from build123d import *

# Parameters (mm, degrees)
F0_W          = 152.4
F0_H          = 15.24
F1_DEPTH      = 12.7
F2_T1_DEPTH   = 190.5
F4_W          = 25.0697992742
F4_H          = 11.7348134518
F5_DEPTH      = 12.7
F5_DEPTH_BACK = 12.7
F7_DEPTH      = 7.62
F7_DEPTH_BACK = 7.62
F8_W          = 65.6082034111
F8_H          = 914.4
F9_DEPTH      = 5.08
F9_DEPTH_BACK = 5.08
F11_DEPTH     = 914.4
F12_DEPTH     = 12.7
F16_R         = 5.08


# Not quite as in the source:
# - a fillet or chamfer that OpenCascade refuses, or shapes differently, is made with other operations: its cross-section is extruded or revolved along the edge and cut away or added


with BuildPart() as f1:
    # F0 (on Right) → F1 (new body)
    with BuildSketch(Plane.YZ):
        with Locations((76.2, -7.62)):
            Rectangle(F0_W, F0_H)
    extrude(amount=F1_DEPTH)

    # F2: fillet of radius 7.62 on 4 edges, made by hand

    # F2_s2 → F2_t1 (cut)
    with BuildSketch(Plane.XZ.offset(-171.45)):
        with BuildLine():
            ThreePointArc((7.62, 0), (2.2318463274, -2.2318463274), (0, -7.62))
            Line((0, -7.62), (0, 0))
            Line((0, 0), (7.62, 0))
        make_face()
        with BuildLine():
            ThreePointArc((7.62, -15.24), (2.2318463274, -13.0081536726), (0, -7.62))
            Line((0, -7.62), (0, -15.24))
            Line((0, -15.24), (7.62, -15.24))
        make_face()
        with BuildLine():
            ThreePointArc((5.08, 0), (10.4681536726, -2.2318463274), (12.7, -7.62))
            Line((12.7, -7.62), (12.7, 0))
            Line((12.7, 0), (5.08, 0))
        make_face()
        with BuildLine():
            ThreePointArc((5.08, -15.24), (10.4681536726, -13.0081536726), (12.7, -7.62))
            Line((12.7, -7.62), (12.7, -15.24))
            Line((12.7, -15.24), (5.08, -15.24))
        make_face()
    extrude(amount=F2_T1_DEPTH, mode=Mode.SUBTRACT)

    # F4 (on offset) → F5 (join, two sides)
    with BuildSketch(Plane.XY.offset(-7.62)) as f5_sk:
        with Locations((6.0101542622, 157.924503088)):
            Rectangle(F4_W, F4_H)
    extrude(amount=F5_DEPTH)
    extrude(f5_sk.sketch, amount=-F5_DEPTH_BACK)

    # F6 (on offset) → F7 (join, two sides)
    with BuildSketch(Plane.XY.offset(-7.62)) as f7_sk:
        with BuildLine():
            Line((6.3893780661, -0.6641601572), (12.5797659928, -0.6641601572))
            ThreePointArc((12.5797659928, -0.6641601572), (34.2227463889, 6.8879561013), (46.4923181534, 26.2505661817))
            Line((46.4923181534, 26.2505661817), (6.3893780661, 26.2505661817))
            Line((6.3893780661, 26.2505661817), (6.3893780661, -0.6641601572))
        make_face()
        with BuildLine():
            Line((0.1989901393, -0.6641601572), (6.3893780661, -0.6641601572))
            Line((6.3893780661, -0.6641601572), (6.3893780661, 26.2505661817))
            Line((6.3893780661, 26.2505661817), (-33.7397263339, 26.2505661817))
            ThreePointArc((-33.7397263339, 26.2505661817), (-21.4587969692, 6.8812254508), (0.1989901393, -0.6641601572))
        make_face()
    extrude(amount=F7_DEPTH)
    extrude(f7_sk.sketch, amount=-F7_DEPTH_BACK)

    # F8 (on offset) → F9 (join, two sides)
    with BuildSketch(Plane.XY.offset(-7.62)) as f9_sk:
        with Locations((6.5435543656, -446.0204662129)):
            Rectangle(F8_W, F8_H)
    extrude(amount=-F9_DEPTH)
    extrude(f9_sk.sketch, amount=F9_DEPTH_BACK)

    # F10 (on face) → F11 (cut)
    with BuildSketch(Plane.XZ.offset(903.2204662129)):
        Polygon((-26.2605473399, -2.54), (-26.2605473399, -7.62), (-9.2217093514, -2.54), align=None)
        Polygon((-9.2217093514, -12.7), (-26.2605473399, -7.62), (-26.2605473399, -12.7), align=None)
        Polygon((39.3476560712, -7.62), (22.3088180826, -12.7), (39.3476560712, -12.7), align=None)
        Polygon((39.3476560712, -2.54), (22.3088180826, -2.54), (39.3476560712, -7.62), align=None)
    extrude(amount=-F11_DEPTH, mode=Mode.SUBTRACT)

    # F12 (add): a face of the model
    f12_faces = [f1.faces().sort_by_distance(p)[0] for p in [
        (6.3771735992, 14.5847815456, 0),
    ]]
    extrude(f12_faces, amount=-F12_DEPTH)

    # F9_face (on face) → F15 section 0
    with BuildSketch(Plane(origin=(6.5435543656, -903.2204662129, -7.62), x_dir=(1, 0, 0), z_dir=(0, -1, 0)), mode=Mode.PRIVATE) as f15_s0:
        Polygon((-32.8041017056, 0), (-15.765263717, -5.08), (15.765263717, -5.08), (32.8041017056, 0), (15.765263717, 5.08), (-15.765263717, 5.08), align=None)
    loft([f15_s0.sketch, Vertex(6.6463528201, -928.6204662129, -7.5741349719)])

    # F16
    f16_edges = [f1.edges().sort_by_distance(p)[0] for p in [
        (-6.524745, 163.79191, -7.62),
        (-6.524745, 157.924503, 5.08),
        (-6.524745, 152.057096, -7.62),
        (-6.524745, 157.924503, -20.32),
        (6.010154, 152.057096, 5.08),
        (18.545054, 157.924503, 5.08),
        (6.010154, 163.79191, 5.08),
        (18.545054, 163.79191, -7.62),
        (18.545054, 157.924503, -20.32),
        (18.545054, 152.057096, -7.62),
        (6.010154, 152.057096, -20.32),
        (6.010154, 163.79191, -20.32),
    ]]
    fillet(f16_edges, radius=F16_R)


solid = f1.part
Verification items for the finished model (mm, model axes). A direction names the side the tool comes from. Coordinates: 2 decimals unless noted, no trailing zeros. Write each loop counter-clockwise with the first axis right and the second up, starting at its lowest first coordinate (ties: lowest second). Pieces come first, ordered by that corner, then holes. Notation, with made-up numbers: M 82.25,66.5 L 138.25,66.5 A20 cw 138.25,70.5 Z; hole C -17.5,24.5 d8. An arc over 180 degrees is marked long. One line per question, with ' | ' between items.
1) Depth check by flat-ended pin: pin 1 Ø1.3 at (x, z) = (7, -0.5) entering from -Y; pin 2 Ø1.5 at (x, z) = (34, 2) entering from -Y (3 decimals); pin 3 Ø2 at (x, y) = (1.5, -804.5) entering from -Z; pin 4 Ø4 at (x, z) = (33, -6.5) entering from +Y. Enter the tip coordinate at first touch or a pass-through.
Solutions:
pin 1: y = -0.66 | pin 2: through | pin 3: z = -12.7 | pin 4: y = 26.25
2) Sectioned sample at A-A on y = -246.5. Record the cut outline in (x, z).
Solutions:
outline: M -26.26,-7.62 L -9.22,-12.7 L 22.31,-12.7 L 39.35,-7.62 L 22.31,-2.54 L -9.22,-2.54 Z
3) Material ranges on L1, parallel to Y at x = 32, z = -13.5; L2, parallel to Z at x = 2.5, y = -590; L3, parallel to Z at x = -26, y = -130, recorded low to high.
Solutions:
L1: 5.26 to 26.25 | L2: -12.7 to -2.54 | L3: -7.7 to -7.54
4) Access from +Z, -Z, +X, -X, +Y, -Y to the whole of each face (thin tool, end or side, straight path). Record for faces 1 (the face through (30.948, -452.421, -10.124)), 2 (the face through (6, -445, -12.7)), 3 (the face through (-25.495, 10.639, -5.82)), 4 (the face through (-17.6, -452.4, -10.2)), 5 (the face through (6, 16, 0)).
Solutions:
face 1: -Z, +X, -Y | face 2: -Z, +X, -X, -Y | face 3: -X, -Y | face 4: -Z, -X, -Y | face 5: +Z, +X, -X, -Y
